For this review, take the finished solid that the model builds, in its own axes (mm). Face numbers are marked on the shaded views. A direction names the side the tool comes from. Round coordinates to 2 decimals unless told otherwise and drop trailing zeros. Order: outer loops, then holes, each group sorted by start corner. A loop starts at its lowest first (then second) coordinate and runs counter-clockwise, first axis right, second up. Notation, with made-up numbers: M 32,2 L 54,2 A25 ccw 54,39 Z; hole C -2.75,41 d7. An arc over 180 degrees is marked long. Use a Markdown table: item, result.
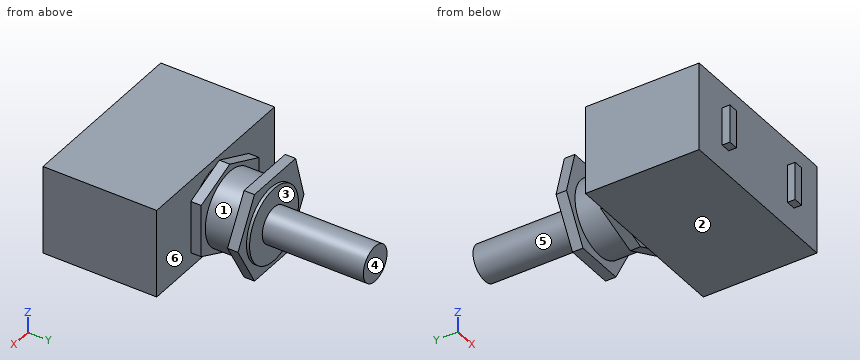
from build123d import *

# Parameters (mm, degrees)
BODYPROFILE_W         = 28.89
BODYPROFILE_H         = 18.5
BODYBOSS_DEPTH        = 7.22
BUSHINGSTEMPROFILE_R  = 6
BUSHINGSTEM_DEPTH     = 9.5
WASHERPROFILE_R       = 6
WASHERBOSS_DEPTH      = 0.6
LOWERNUTBOSS_DEPTH    = 1.7
UPPERNUTBOSS_START    = 5
UPPERNUTBOSS_DEPTH    = 1.7
ACTUATORBASEPROFILE_R = 2.9
ACTUATORBOSS_DEPTH    = 16.45
LEFTTERMINALPROFILE_W = 1.6
LEFTTERMINALPROFILE_H = 6.2
TERMINALBOSSES_DEPTH  = 10.5


with BuildPart() as part:
    # BodyProfile → BodyBoss (new, symmetric)
    with BuildSketch(Plane.XY):
        Rectangle(BODYPROFILE_W, BODYPROFILE_H)
    extrude(amount=BODYBOSS_DEPTH, both=True)

    # BushingStemProfile → BushingStem (add)
    with BuildSketch(Plane(origin=(0, 9.25, 0), x_dir=(1, 0, 0), z_dir=(0, 1, 0))):
        with Locations(Location((0, 0, 0), (0, 0, 270))):
            Circle(BUSHINGSTEMPROFILE_R)
    extrude(amount=BUSHINGSTEM_DEPTH)

    # WasherProfile → WasherBoss (add)
    with BuildSketch(Plane(origin=(0, 9.25, 0), x_dir=(1, 0, 0), z_dir=(0, 1, 0))):
        with Locations(Location((0, 0, 0), (0, 0, 270))):
            Circle(WASHERPROFILE_R)
    extrude(amount=WASHERBOSS_DEPTH)

    # LowerNutProfile → LowerNutBoss (add)
    with BuildSketch(Plane(origin=(0, 9.85, 0), x_dir=(1, 0, 0), z_dir=(0, 1, 0))):
        Polygon((7, 4.0415), (0, 7.22), (-7.181103891, 4.52386712), (-7.181103891, -4.0415), (0, -7.22), (7, -4.515434504), align=None)
    extrude(amount=LOWERNUTBOSS_DEPTH)

    # UpperNutProfile → UpperNutBoss (add)
    with BuildSketch(Plane(origin=(0, 11.55, 0), x_dir=(1, 0, 0), z_dir=(0, 1, 0)).offset(UPPERNUTBOSS_START)):
        Polygon((8.083, 0), (4.0415, 7.22), (-4.0415, 7.22), (-8.083, 0), (-6.045192426, -7.22), (4.0415, -7.22), align=None)
    extrude(amount=UPPERNUTBOSS_DEPTH)

    # ActuatorBaseProfile → ActuatorBoss (add)
    with BuildSketch(Plane(origin=(0, 18.75, 0), x_dir=(1, 0, 0), z_dir=(0, 1, 0))):
        with Locations(Location((0, 0, 0), (0, 0, 270))):
            Circle(ACTUATORBASEPROFILE_R)
    extrude(amount=ACTUATORBOSS_DEPTH)

    # LeftTerminalProfile → TerminalBosses (add)
    with BuildSketch(Plane(origin=(0, 0, 0), x_dir=(1, 0, 0), z_dir=(0, 1, 0))):
        with Locations((-8, 0)):
            Rectangle(LEFTTERMINALPROFILE_W, LEFTTERMINALPROFILE_H)
        with Locations((8, 0)):
            Rectangle(LEFTTERMINALPROFILE_W, LEFTTERMINALPROFILE_H)
    extrude(amount=-TERMINALBOSSES_DEPTH)


solid = part.part
Q1. Add section C-C (y = 32). Write out the cut boundary in (x, z).
Determined:
| item | result |
|---|---|
| outline | C 0,0 d5.8 |
Q2. Draft analysis for pull direction Y (two halves, no side actions). For the marked faces 4, 5 and 6, state which applies: pulls with the +Y half, pulls with the -Y half, needs draft (parallel to the pull), parting line crosses it, or undercut.
Determined:
| item | result |
|---|---|
| face 4 | pulls with the +Y half |
| face 5 | needs draft |
| face 6 | undercut |
Q3. Machinability: for the marked faces 1, 2 and 3, which of the approach directions +Z, -Z, +X, -X, +Y, -Y give a long, thin tool a straight path to every point of the face, cutting with its end or side? Answer none if there is none.
Determined:
| item | result |
|---|---|
| face 1 | none |
| face 2 | -Z, +X, -X, +Y, -Y |
| face 3 | +Y |
Q4. Clearance check with flat-ended pins moving along their axes: pin 1 (3 mm diameter, centred on y = 28, z = -3.5, fed in from +X); pin 2 (1.4 mm diameter, centred on y = -10, z = 0, fed in from -X); pin 3 (0.8 mm diameter, centred on y = 10.5, z = 0, fed in from +X). State where each tip first meets the part, or that it passes through.
Determined:
| item | result |
|---|---|
| pin 1 | stops at x = 2.1 |
| pin 2 | stops at x = -8.8 |
| pin 3 | stops at x = 7 |
Q5. Wall thickness on line 1 along Y through (x, z) = (-1.75, -6.5); line 2 along Y through (x, z) = (5.25, 2); line 3 along X through (y, z) = (10, 0): over which ranges is each line inside the solid? List them lowest first. Write a range as [from, to].
Determined:
| item | result |
|---|---|
| line 1 | y = [-9.25, 9.25], [9.85, 11.55], [16.55, 18.25] |
| line 2 | y = [-9.25, 18.75] |
| line 3 | x = [-7.18, 7] |
Q6. Add section D-D (x = 9.5). Write out the cut boundary in (y, z).
Determined:
| item | result |
|---|---|
| outline | M -9.25,-7.22 L 9.25,-7.22 L 9.25,7.22 L -9.25,7.22 Z |
Q7. Add section B-B (z = 5.5). Write out the cut boundary in (x, y) (3 decimals), then the cut area to 3 significant figures.
Determined:
| item | result |
|---|---|
| outline | M -14.445,-9.25 L 14.445,-9.25 L 14.445,9.25 L 2.398,9.25 L 2.398,9.85 L 4.452,9.85 L 4.452,11.55 L 2.398,11.55 L 2.398,16.55 L 5.004,16.55 L 5.004,18.25 L 2.398,18.25 L 2.398,18.75 L -2.398,18.75 L -2.398,18.25 L -6.531,18.25 L -6.531,16.55 L -2.398,16.55 L -2.398,11.55 L -3.886,11.55 L -3.886,9.85 L -2.398,9.85 L -2.398,9.25 L -14.445,9.25 Z |
| area | 598 mm^2 |
Q8. Add section A-A (x = 5.5). Write out the cut boundary in (y, z).
Determined:
| item | result |
|---|---|
| outline | M -9.25,-7.22 L 9.25,-7.22 L 9.25,-2.4 L 9.85,-2.4 L 9.85,-4.72 L 11.55,-4.72 L 11.55,-2.4 L 16.55,-2.4 L 16.55,-4.61 L 18.25,-4.61 L 18.25,-2.4 L 18.75,-2.4 L 18.75,2.4 L 18.25,2.4 L 18.25,4.61 L 16.55,4.61 L 16.55,2.4 L 11.55,2.4 L 11.55,5.09 L 9.85,5.09 L 9.85,2.4 L 9.25,2.4 L 9.25,7.22 L -9.25,7.22 Z |
